Read the model definition and answer for the solid it produces. Units are mm, in the model's axes. Face numbers are marked on the shaded views. A direction names the side the tool comes from. Round coordinates to 2 decimals unless told otherwise and drop trailing zeros. Write each loop counter-clockwise with the first axis right and the second up, starting at its lowest first coordinate (ties: lowest second). Pieces come first, ordered by that corner, then holes. Notation, with made-up numbers: (20.25, -19) - (74.25, -19) arc R23 ccw to (74.25, -7) - close; hole circle Ø2 at (6.25, 54). An arc over 180 degrees is marked (long way). Answer as CSV lines item,"result". Start each with the question number.
1) This flat-tipped pin is pushed along its axis until it touches: pin 1 (1 mm diameter, centred on x = 22, y = -117, fed in from +Z). Where does it stop, or does it pass through?
2) Find section A-A on z = 36. Determine the outline of the cut face in (x, y).
3) Consider line 1 along X through (y, z) = (-7, 6); line 2 along Z through (x, y) = (5.75, -88). Determine where each line is inside the solid, lowest interval first.
4) For a pull along X with two mould halves and no side action, classify the marked faces 1, 2 and 3 as +X half, -X half, draft (parallel to the pull), parting line (faces both ways), or undercut.
5) Find section C-C on x = 8.5. Determine the outline of the cut face in (y, z), then the cut area to 3 significant figures.
6) Which of the six approach directions +Z, -Z, +X, -X, +Y, -Y give full straight-line access (tool end or side, diameter ignored) to the marked faces 4 and 5?
7) Find section B-B on y = -46. Determine the outline of the cut face in (x, z), then the cut area to 3 significant figures.
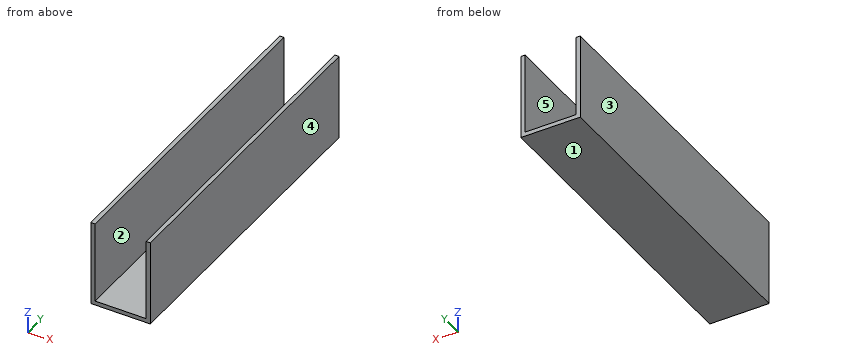
from build123d import *

# Parameters (mm, degrees)
F0_W     = 28.999942
F0_H     = 41.91
F1_DEPTH = 155.999942
F2_W     = 24.892
F2_H     = 39.878
F3_DEPTH = 156.000942


with BuildPart() as f1:
    # F0 (on Front) → F1 (new body)
    with BuildSketch(Plane.XZ):
        with Locations((14.499971, 20.955)):
            Rectangle(F0_W, F0_H)
    extrude(amount=F1_DEPTH)

    # F2 (on face) → F3 (cut, through all)
    with BuildSketch(Plane(origin=(0, 0, 0), x_dir=(-1, 0, 0), z_dir=(0, 1, 0))):
        with Locations((-14.521942, 21.971)):
            Rectangle(F2_W, F2_H)
    extrude(amount=-F3_DEPTH, mode=Mode.SUBTRACT)


solid = f1.part
Check values:
1,pin 1,"stops at z = 2.03"
2,outline,"(0, -156) - (2.08, -156) - (2.08, 0) - (0, 0) - close; (26.97, -156) - (29, -156) - (29, 0) - (26.97, 0) - close"
3,line 1,"x = 0 to 2.08, 26.97 to 29"
3,line 2,"z = 0 to 2.03"
4,face 1,"draft"
4,face 2,"undercut"
4,face 3,"-X half"
5,outline,"(-156, 0) - (0, 0) - (0, 2.03) - (-156, 2.03) - close"
5,area,"317 mm^2"
6,face 4,"+Z, -Z, +X, +Y, -Y"
6,face 5,"+Z, +Y, -Y"
7,outline,"(0, 0) - (29, 0) - (29, 41.91) - (26.97, 41.91) - (26.97, 2.03) - (2.08, 2.03) - (2.08, 41.91) - (0, 41.91) - close"
7,area,"223 mm^2"
